```python
from build123d import *

# Parameters (mm, degrees)
MODEL_R                 = 1.5
MODEL_W                 = 3
MODEL_H                 = 3
SALIENTE_EXTRUIR1_DEPTH = 3


with BuildPart() as part:
    # Model → Saliente-Extruir1 (new body)
    with BuildSketch(Plane.XY):
        with BuildLine():
            Line((20.979107628, 285.503511394), (19.979107628, 286.503511394))
            Line((19.979107628, 286.503511394), (20.979107628, 287.503511394))
            Line((20.979107628, 287.503511394), (25.479107628, 287.503511394))
            ThreePointArc((25.479107628, 287.503511394), (28.661088143, 286.185491909), (29.979107628, 283.003511394))
            Line((29.979107628, 283.003511394), (29.979107628, 273.910365643))
            Line((29.979107628, 273.910365643), (38.532408487, 265.357064784))
            ThreePointArc((38.532408487, 265.357064784), (38.971748315, 264.296404613), (38.532408487, 263.235744441))
            Line((38.532408487, 263.235744441), (33.950301706, 258.65363766))
            ThreePointArc((33.950301706, 258.65363766), (33.510961878, 257.592977488), (33.950301706, 256.532317316))
            Line((33.950301706, 256.532317316), (47.5397678, 242.942851222))
            ThreePointArc((47.5397678, 242.942851222), (48.026402823, 242.617692095), (48.600427972, 242.503511394))
            Line((48.600427972, 242.503511394), (52.479107628, 242.503511394))
            ThreePointArc((52.479107628, 242.503511394), (56.979107628, 238.003511394), (52.479107628, 233.503511394))
            Line((52.479107628, 233.503511394), (25.479107628, 233.503511394))
            ThreePointArc((25.479107628, 233.503511394), (22.297127113, 234.821530879), (20.979107628, 238.003511394))
            Line((20.979107628, 238.003511394), (20.979107628, 239.503511394))
            Line((20.979107628, 239.503511394), (19.979107628, 240.503511394))
            Line((19.979107628, 240.503511394), (20.979107628, 241.503511394))
            Line((20.979107628, 241.503511394), (19.979107628, 242.503511394))
            Line((19.979107628, 242.503511394), (20.979107628, 243.503511394))
            Line((20.979107628, 243.503511394), (19.979107628, 244.503511394))
            Line((19.979107628, 244.503511394), (20.979107628, 245.503511394))
            Line((20.979107628, 245.503511394), (19.979107628, 246.503511394))
            Line((19.979107628, 246.503511394), (20.979107628, 247.503511394))
            Line((20.979107628, 247.503511394), (19.979107628, 248.503511394))
            Line((19.979107628, 248.503511394), (20.979107628, 249.503511394))
            Line((20.979107628, 249.503511394), (19.979107628, 250.503511394))
            Line((19.979107628, 250.503511394), (20.979107628, 251.503511394))
            Line((20.979107628, 251.503511394), (19.979107628, 252.503511394))
            Line((19.979107628, 252.503511394), (20.979107628, 253.503511394))
            Line((20.979107628, 253.503511394), (19.979107628, 254.503511394))
            Line((19.979107628, 254.503511394), (20.979107628, 255.503511394))
            Line((20.979107628, 255.503511394), (19.979107628, 256.503511394))
            Line((19.979107628, 256.503511394), (20.979107628, 257.503511394))
            Line((20.979107628, 257.503511394), (19.979107628, 258.503511394))
            Line((19.979107628, 258.503511394), (20.979107628, 259.503511394))
            Line((20.979107628, 259.503511394), (19.979107628, 260.503511394))
            Line((19.979107628, 260.503511394), (20.979107628, 261.503511394))
            Line((20.979107628, 261.503511394), (19.979107628, 262.503511394))
            Line((19.979107628, 262.503511394), (20.979107628, 263.503511394))
            Line((20.979107628, 263.503511394), (19.979107628, 264.503511394))
            Line((19.979107628, 264.503511394), (20.979107628, 265.503511394))
            Line((20.979107628, 265.503511394), (19.979107628, 266.503511394))
            Line((19.979107628, 266.503511394), (20.979107628, 267.503511394))
            Line((20.979107628, 267.503511394), (19.979107628, 268.503511394))
            Line((19.979107628, 268.503511394), (20.979107628, 269.503511394))
            Line((20.979107628, 269.503511394), (19.979107628, 270.503511394))
            Line((19.979107628, 270.503511394), (20.979107628, 271.503511394))
            Line((20.979107628, 271.503511394), (19.979107628, 272.503511394))
            Line((19.979107628, 272.503511394), (20.979107628, 273.503511394))
            Line((20.979107628, 273.503511394), (19.979107628, 274.503511394))
            Line((19.979107628, 274.503511394), (20.979107628, 275.503511394))
            Line((20.979107628, 275.503511394), (19.979107628, 276.503511394))
            Line((19.979107628, 276.503511394), (20.979107628, 277.503511394))
            Line((20.979107628, 277.503511394), (19.979107628, 278.503511394))
            Line((19.979107628, 278.503511394), (20.979107628, 279.503511394))
            Line((20.979107628, 279.503511394), (19.979107628, 280.503511394))
            Line((19.979107628, 280.503511394), (20.979107628, 281.503511394))
            Line((20.979107628, 281.503511394), (19.979107628, 282.503511394))
            Line((19.979107628, 282.503511394), (20.979107628, 283.503511394))
            Line((20.979107628, 283.503511394), (19.979107628, 284.503511394))
            Line((19.979107628, 284.503511394), (20.979107628, 285.503511394))
        make_face()
        with Locations((43.479107628, 238.003511394)):
            Circle(MODEL_R, mode=Mode.SUBTRACT)
        with Locations((34.479107628, 238.003511394)):
            Circle(MODEL_R, mode=Mode.SUBTRACT)
        with Locations((52.479107628, 238.003511394)):
            Circle(MODEL_R, mode=Mode.SUBTRACT)
        with Locations((25.479107628, 238.003511394)):
            Circle(MODEL_R, mode=Mode.SUBTRACT)
        with Locations((25.479107628, 283.003511394)):
            Rectangle(MODEL_W, MODEL_H, mode=Mode.SUBTRACT)
        with Locations((25.479107628, 247.003511394)):
            Rectangle(MODEL_W, MODEL_H, mode=Mode.SUBTRACT)
        with Locations((25.479107628, 274.003511394)):
            Rectangle(MODEL_W, MODEL_H, mode=Mode.SUBTRACT)
        with Locations((25.479107628, 256.003511394)):
            Rectangle(MODEL_W, MODEL_H, mode=Mode.SUBTRACT)
        with Locations((25.479107628, 265.003511394)):
            Rectangle(MODEL_W, MODEL_H, mode=Mode.SUBTRACT)
        with Locations((34.479107628, 247.003511394)):
            Rectangle(MODEL_W, MODEL_H, mode=Mode.SUBTRACT)
        with BuildLine():
            Line((36.057534753, 263.235744441), (34.820097886, 261.998307574))
            ThreePointArc((34.820097886, 261.998307574), (34.2897678, 261.77863766), (33.759437714, 261.998307574))
            Line((33.759437714, 261.998307574), (30.223903808, 265.53384148))
            ThreePointArc((30.223903808, 265.53384148), (30.004233894, 266.064171566), (30.223903808, 266.594501652))
            Line((30.223903808, 266.594501652), (31.461340675, 267.831938519))
            ThreePointArc((31.461340675, 267.831938519), (31.991670761, 268.051608433), (32.522000847, 267.831938519))
            Line((32.522000847, 267.831938519), (36.057534753, 264.296404613))
            ThreePointArc((36.057534753, 264.296404613), (36.277204667, 263.766074527), (36.057534753, 263.235744441))
        make_face(mode=Mode.SUBTRACT)
    extrude(amount=SALIENTE_EXTRUIR1_DEPTH)


solid = part.part
```
Design review of the part built by this model. Coordinates are the model's own, in mm. A direction names the side the tool comes from. Coordinates: 2 decimals unless noted, no trailing zeros. Loops run counter-clockwise (first coordinate to the right, second up) from the corner with the lowest first, then second, coordinate; pieces in that order, holes last. Notation, with made-up numbers: (-25, 70) - (15, 70) arc R20 ccw to (15, 80) - close; hole circle Ø3 at (-16, 24.5). An arc over 180 degrees is marked (long way). Use CSV: the item, a comma, the result in double quotes. Start each with the question number.
1) Wall thickness on L1, parallel to X at y = 282, z = 0.6; L2, parallel to Y at x = 37.5, z = 1.75; L3, parallel to X at y = 273, z = 2.7: over which ranges is each line inside the solid? List them lowest first. Write a range as from..to.
2) For pin 1 Ø0.9 at (y, z) = (264.5, 1) entering from +X; pin 2 Ø3 at (x, y) = (40, 247) entering from -Z; pin 3 Ø1 at (y, z) = (259, 1) entering from +X; pin 4 Ø0.9 at (y, z) = (283, 2) entering from +X, all flat-tipped, find the tip position at first contact; note any pin that passes through.
3) Consider section A-A on z = 1.2. Give the number of separate pieces and of enclosed holes in the cut face, then the cut area to 3 significant figures.
4) Consider section C-C on x = 55. Write out the cut boundary in (y, z), then the cut area to 3 significant figures.
5) Tool access review of faces 4 (the flat face through (25, 254.504, 1)), 5 (the flat face through (20.486, 255.997, 1.479)), 6 (the flat face through (36.273, 260.977, 1.479)), 7 (the flat face through (29.979, 279, 1)): name each direction out of +Z, -Z, +X, -X, +Y, -Y from which nothing blocks a thin tool from reaching the whole face with its end or side.
6) Consider section B-B on x = 49.5. Write out the cut boundary in (y, z).
7) The part is to be moulded in two halves that separate along X. For faces 1 (the flat face through (23, 287.504, 1)), 2 (the cylindrical face through (28.626, 286.22, 1.479)), 3 (the flat face through (25, 284.504, 1)), say which applies: +X half, -X half, draft (parallel to the pull), parting line (faces both ways), or undercut.
Geometry says:
1,L1,"20.48..23.98, 26.98..29.98"
1,L2,"233.5..252.98, 262.2..266.39"
1,L3,"20.48..23.98, 26.98..30.89"
2,pin 1,"x = 38.97"
2,pin 2,"z = 0"
2,pin 3,"x = 34.8"
2,pin 4,"x = 29.98"
3,separate pieces,"1"
3,enclosed holes,"11"
3,area,"879 mm^2"
4,outline,"(234.28, 0) - (241.73, 0) - (241.73, 3) - (234.28, 3) - close"
4,area,"22.4 mm^2"
5,face 4,"+Z, -Z"
5,face 5,"+Z, -Z, -X"
5,face 6,"+Z, -Z, +X"
5,face 7,"+Z, -Z, +X, +Y"
6,outline,"(233.5, 0) - (242.5, 0) - (242.5, 3) - (233.5, 3) - close"
7,face 1,"draft"
7,face 2,"+X half"
7,face 3,"undercut"
